Drawing for the job (mm, zero at the part's lowest x, y, z). A direction names the side the tool comes from. Give positions to 0.01 mm unless a question says otherwise; leave off trailing zeros. Order: outer loops, then holes, each group sorted by start corner. A loop starts at its lowest first (then second) coordinate and runs counter-clockwise, first axis right, second up. Notation, with made-up numbers: (64.5, 31.5) -> (104.5, 31.5) arc R12 cw to (104.5, 50.5) -> close; hole circle Ø7 at (42, -25). An arc over 180 degrees is marked (long way). One line per item, written item: value. Start each with the question number.
(1) Which spindle directions (+Z, -Z, +X, -X, +Y, -Y) get a long thin tool onto all of the face, cutting with end or side? Do the marked faces 5 and 6. Say none if no direction does.
(2) Saw through at D-D on y = 12.75. Give the cut face in (x, z), plus the area to 3 significant figures.
(3) Saw through at C-C on z = 1.9. Give the cut face in (x, y), plus the area to 3 significant figures.
(4) Probe line 1 (X direction, y = 12, z = 3.8); line 2 (Y direction, x = 8.25, z = 0.8). List the from-to ranges inside material, lowest first.
(5) Pin check, flat tip, straight feed: pin 1 (1 mm diameter, centred on x = 12.5, y = 11, fed in from -Z). Stop position of the tip, or through.
(6) Saw through at A-A on x = 7.25. Give the cut face in (y, z), plus the area to 3 significant figures.
(7) Two-plate mould, pull along Y, no slides. Class the marked faces 1, 2, 3 and 4: +Y half, -Y half, draft (parallel to the pull), parting line (faces both ways), or undercut.
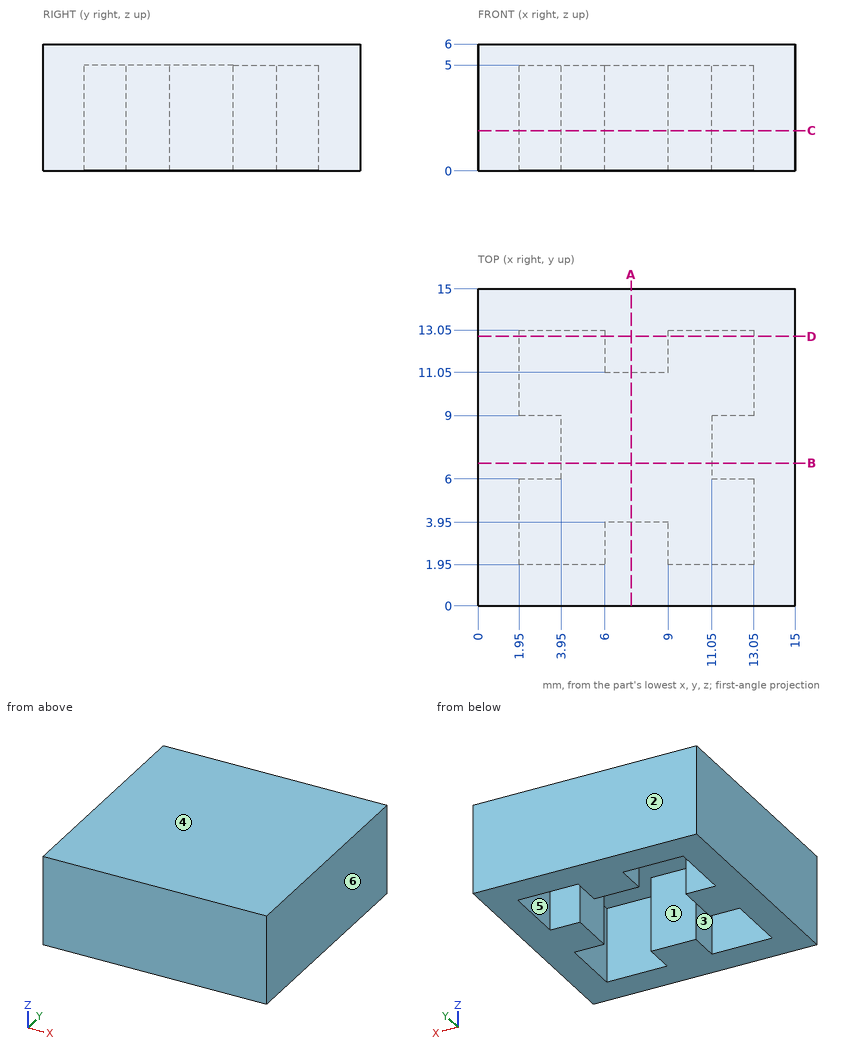
Results below:
1. face 5: -Z
1. face 6: +Z, -Z, +X, +Y, -Y
2. outline: (0, 0) -> (1.95, 0) -> (1.95, 5) -> (6, 5) -> (6, 0) -> (9, 0) -> (9, 5) -> (13.05, 5) -> (13.05, 0) -> (15, 0) -> (15, 6) -> (0, 6) -> close
2. area: 49.5 mm²
3. outline: (0, 0) -> (15, 0) -> (15, 15) -> (0, 15) -> close; hole (1.95, 1.95) -> (6, 1.95) -> (6, 3.95) -> (9, 3.95) -> (9, 1.95) -> (13.05, 1.95) -> (13.05, 6) -> (11.05, 6) -> (11.05, 9) -> (13.05, 9) -> (13.05, 13.05) -> (9, 13.05) -> (9, 11.05) -> (6, 11.05) -> (6, 13.05) -> (1.95, 13.05) -> (1.95, 9) -> (3.95, 9) -> (3.95, 6) -> (1.95, 6) -> close
3. area: 126 mm²
4. line 1: x = 0 to 1.95, 6 to 9, 13.05 to 15
4. line 2: y = 0 to 3.95, 11.05 to 15
5. pin 1: stops at z = 5
6. outline: (0, 0) -> (3.95, 0) -> (3.95, 5) -> (11.05, 5) -> (11.05, 0) -> (15, 0) -> (15, 6) -> (0, 6) -> close
6. area: 54.5 mm²
7. face 1: undercut
7. face 2: +Y half
7. face 3: undercut
7. face 4: draft
